from build123d import *

# Parameters (mm, degrees)
SCHIZZO1_R                     = 13.03
ESTRUSIONE_ESTRUSIONE1_DEPTH   = 2.93
SCHIZZO2_R                     = 3.575
ESTRUSIONE_ESTRUSIONE2_DEPTH   = 0.86
SCHIZZO3_R                     = 4.725
ESTRUSIONE_ESTRUSIONE3_DEPTH   = 4.31
SCHIZZO4_R                     = 2.5
TAGLIO_ESTRUSIONE1_DEPTH       = 21.12887975
FORO_FILETTATO_M3X0_5_1_D      = 2.5
TAGLIO_ESTRUSIONE2_DEPTH       = 2.1
FORO_FILETTATO_M3X0_5_2_REACH  = 25.201
FORO_FILETTATO_M3X0_5_2_BORE_R = 1.25


with BuildPart() as part:
    # Schizzo1 → Estrusione-Estrusione1 (new body)
    with BuildSketch(Plane.XY):
        with Locations(Location((0, 0, 0), (0, 0, 180))):
            Circle(SCHIZZO1_R)
    extrude(amount=ESTRUSIONE_ESTRUSIONE1_DEPTH)

    # Schizzo2 → Estrusione-Estrusione2 (add)
    with BuildSketch(Plane.XY.offset(2.93)):
        Circle(SCHIZZO2_R)
    extrude(amount=ESTRUSIONE_ESTRUSIONE2_DEPTH)

    # Schizzo3 → Estrusione-Estrusione3 (add)
    with BuildSketch(Plane(origin=(0, 0, 0), x_dir=(-1, 0, 0), z_dir=(0, 0, -1))):
        with Locations(Location((0, 0, 0), (0, 0, 180))):
            Circle(SCHIZZO3_R)
    extrude(amount=ESTRUSIONE_ESTRUSIONE3_DEPTH)

    # Schizzo4 → Taglio-Estrusione1 (cut, through all)
    with BuildSketch(Plane(origin=(0, 0, -4.31), x_dir=(-1, 0, 0), z_dir=(0, 0, -1))):
        Circle(SCHIZZO4_R)
    extrude(amount=-TAGLIO_ESTRUSIONE1_DEPTH, mode=Mode.SUBTRACT)

    # Foro filettato M3x0.5-1 (through all)
    with Locations(Plane.XY.offset(2.93)):
        with Locations((0, 8), (0, -8), (8, 0), (-8, 0)):
            Hole(FORO_FILETTATO_M3X0_5_1_D / 2)

    # Schizzo7 → Taglio-Estrusione2 (cut)
    with BuildSketch(Plane(origin=(0, 0, 0), x_dir=(-1, 0, 0), z_dir=(0, 0, -1))):
        with BuildLine():
            Line((2.675, 9.38083152), (2.675, 5.839895119))
            ThreePointArc((2.675, 5.839895119), (2.799611887, 5.356474337), (3.142391304, 4.993533507))
            ThreePointArc((3.142391304, 4.993533507), (4.171930009, 4.171930009), (4.993533507, 3.142391304))
            ThreePointArc((4.993533507, 3.142391304), (5.356474337, 2.799611887), (5.839895119, 2.675))
            Line((5.839895119, 2.675), (9.38083152, 2.675))
            ThreePointArc((9.38083152, 2.675), (10.206895763, 3.111424037), (10.311931422, 4.039764268))
            ThreePointArc((10.311931422, 4.039764268), (7.831207602, 7.831207602), (4.039764268, 10.311931422))
            ThreePointArc((4.039764268, 10.311931422), (3.111424037, 10.206895763), (2.675, 9.38083152))
        make_face()
        with BuildLine():
            Line((-2.675, 9.38083152), (-2.675, 5.839895119))
            ThreePointArc((-2.675, 5.839895119), (-2.799611887, 5.356474337), (-3.142391304, 4.993533507))
            ThreePointArc((-3.142391304, 4.993533507), (-4.171930009, 4.171930009), (-4.993533507, 3.142391304))
            ThreePointArc((-4.993533507, 3.142391304), (-5.356474337, 2.799611887), (-5.839895119, 2.675))
            Line((-5.839895119, 2.675), (-9.38083152, 2.675))
            ThreePointArc((-9.38083152, 2.675), (-10.206895763, 3.111424037), (-10.311931422, 4.039764268))
            ThreePointArc((-10.311931422, 4.039764268), (-7.831207602, 7.831207602), (-4.039764268, 10.311931422))
            ThreePointArc((-4.039764268, 10.311931422), (-3.111424037, 10.206895763), (-2.675, 9.38083152))
        make_face()
        with BuildLine():
            Line((9.38083152, -2.675), (5.839895119, -2.675))
            ThreePointArc((5.839895119, -2.675), (5.356474337, -2.799611887), (4.993533507, -3.142391304))
            ThreePointArc((4.993533507, -3.142391304), (4.171930009, -4.171930009), (3.142391304, -4.993533507))
            ThreePointArc((3.142391304, -4.993533507), (2.799611887, -5.356474337), (2.675, -5.839895119))
            Line((2.675, -5.839895119), (2.675, -9.38083152))
            ThreePointArc((2.675, -9.38083152), (3.111424037, -10.206895763), (4.039764268, -10.311931422))
            ThreePointArc((4.039764268, -10.311931422), (7.831207602, -7.831207602), (10.311931422, -4.039764268))
            ThreePointArc((10.311931422, -4.039764268), (10.206895763, -3.111424037), (9.38083152, -2.675))
        make_face()
        with BuildLine():
            Line((-2.675, -9.38083152), (-2.675, -5.839895119))
            ThreePointArc((-2.675, -5.839895119), (-2.799611887, -5.356474337), (-3.142391304, -4.993533507))
            ThreePointArc((-3.142391304, -4.993533507), (-4.171930009, -4.171930009), (-4.993533507, -3.142391304))
            ThreePointArc((-4.993533507, -3.142391304), (-5.356474337, -2.799611887), (-5.839895119, -2.675))
            Line((-5.839895119, -2.675), (-9.38083152, -2.675))
            ThreePointArc((-9.38083152, -2.675), (-10.206895763, -3.111424037), (-10.311931422, -4.039764268))
            ThreePointArc((-10.311931422, -4.039764268), (-7.831207602, -7.831207602), (-4.039764268, -10.311931422))
            ThreePointArc((-4.039764268, -10.311931422), (-3.111424037, -10.206895763), (-2.675, -9.38083152))
        make_face()
    extrude(amount=-TAGLIO_ESTRUSIONE2_DEPTH, mode=Mode.SUBTRACT)

    # Foro filettato M3x0.5-2 bore → Foro filettato M3x0.5-2 (cut, up to next)
    with BuildSketch(Plane(origin=(4.440047633, -1.616045177, 0), x_dir=(-0.3420201433256662, -0.9396926207859093, 0), z_dir=(0.9396926207859093, -0.3420201433256662, 0)), mode=Mode.PRIVATE) as foro_filettato_m3x0_5_2_sk1:
        with Locations((0, 2.155)):
            Circle(FORO_FILETTATO_M3X0_5_2_BORE_R)
    foro_filettato_m3x0_5_2_tool1 = extrude(foro_filettato_m3x0_5_2_sk1.sketch, amount=-FORO_FILETTATO_M3X0_5_2_REACH, mode=Mode.PRIVATE) & part.part
    add(foro_filettato_m3x0_5_2_tool1.solids().sort_by_distance((4.440048, -1.616045, -2.155))[0], mode=Mode.SUBTRACT)


solid = part.part
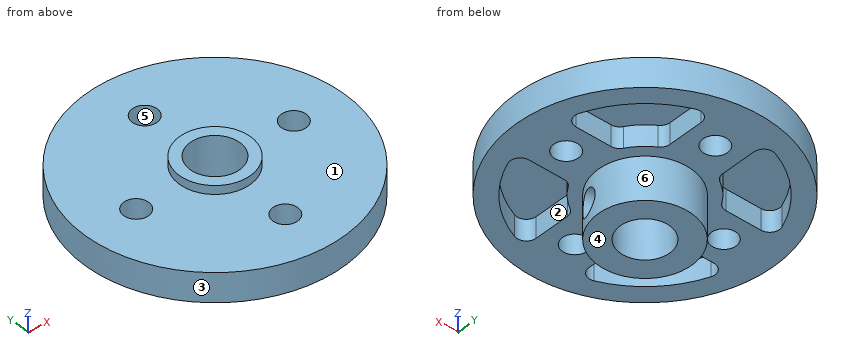
CAD build for the part. Positions are in the model's coordinates, mm. Face numbers are marked on the shaded views. A direction names the side the tool comes from. Round coordinates to 2 decimals unless told otherwise and drop trailing zeros. Loops run counter-clockwise (first coordinate to the right, second up) from the corner with the lowest first, then second, coordinate; pieces in that order, holes last. Notation, with made-up numbers: M -37,-5.75 L 15,-5.75 A26 ccw 15,19.25 Z; hole C 52.5,44.5 d11. An arc over 180 degrees is marked long. One line per question, with ' | ' between items. Start each with the question number.
Item 1: Wall check: line 1 (Y direction, x = 0, z = 1.5); line 2 (Y direction, x = 0, z = -1.25) (3 decimals); line 3 (Y direction, x = 8, z = 1.5) (3 decimals). Give the ranges that are in metal, low to high.
Item 2: Pin check, flat tips, straight feed: pin 1 Ø2.5 at (x, y) = (7, -6.5) entering from -Z; pin 2 Ø2 at (x, y) = (9.5, -10) entering from +Z; pin 3 Ø2.5 at (x, z) = (8, 0.5) entering from -Y; pin 4 Ø1.5 at (x, y) = (0, -8) entering from +Z. Stop position of each tip, or through.
Item 3: Cut at C-C, the plane z = -0.5. Write the cut outline in (x, y) (3 decimals).
Item 4: Cut at A-A, the plane x = 0. Write the cut outline in (y, z) (3 decimals), plus the area to 3 significant figures.
Item 5: Cut at D-D, the plane y = 10. Write the cut outline in (x, z).
Item 6: Which spindle directions (+Z, -Z, +X, -X, +Y, -Y) get a long thin tool onto all of the face, cutting with end or side? Do the marked faces 1, 2 and 3. Say none if no direction does.
Item 7: Two-plate mould, pull along Y, no slides. Class the marked faces 4, 5 and 6: pulls with the +Y half, pulls with the -Y half, needs draft (parallel to the pull), parting line crosses it, or undercut.
Item 8: Cut at B-B, the plane x = 7.5. Write the cut outline in (y, z) (3 decimals), plus the area to 3 significant figures.
Responses:
1) line 1: y = -13.03 to -9.25, -6.75 to -2.5, 2.5 to 6.75, 9.25 to 13.03 | line 2: y = -4.725 to -2.5, 2.5 to 4.725 | line 3: y = -10.285 to -7.659, -2.675 to -1.25, 1.25 to 2.675, 7.659 to 10.285
2) pin 1: stops at z = 2.1 | pin 2: stops at z = 2.93 | pin 3: stops at y = -11.15 | pin 4: passes through
3) outline: C 0,0 d9.45; hole C 0,0 d5
4) outline: M -13.03,0 L -9.25,0 L -9.25,2.93 L -13.03,2.93 Z; M -6.75,0 L -4.725,0 L -4.725,-4.31 L -2.5,-4.31 L -2.5,3.79 L -3.575,3.79 L -3.575,2.93 L -6.75,2.93 Z; M 2.5,-4.31 L 4.725,-4.31 L 4.725,0 L 6.75,0 L 6.75,2.93 L 3.575,2.93 L 3.575,3.79 L 2.5,3.79 Z; M 9.25,0 L 13.03,0 L 13.03,2.93 L 9.25,2.93 Z | area: 68.1 mm²
5) outline: M -8.35,0 L -4.76,0 L -4.76,2.1 L -2.89,2.1 L -2.89,0 L 2.89,0 L 2.89,2.1 L 4.76,2.1 L 4.76,0 L 8.35,0 L 8.35,2.93 L -8.35,2.93 Z
6) face 1: +Z | face 2: -Z | face 3: +Z, -Z
7) face 4: needs draft | face 5: undercut | face 6: parting line crosses it
8) outline: M -10.655,0 L -8.149,0 L -8.149,2.1 L -2.675,2.1 L -2.675,0 L -1.146,0 L -1.146,2.93 L -10.655,2.93 Z; M 1.146,0 L 2.675,0 L 2.675,2.1 L 8.149,2.1 L 8.149,0 L 10.655,0 L 10.655,2.93 L 1.146,2.93 Z | area: 32.7 mm²
